Input: part model. Units: mm. Frame: model coordinates. A direction names the side the tool comes from. Give positions to 0.01 mm unless a question says otherwise; leave off trailing zeros. Write each loop counter-clockwise with the first axis right and the second up, starting at its lowest first coordinate (ties: lowest second). Pieces come first, ordered by that corner, then holes. Notation, with made-up numbers: (75.5, 51.25) - (97.5, 51.25) arc R16 cw to (97.5, 60.25) - close; hole circle Ø4 at (-14.75, 69.5). An arc over 180 degrees is marked (long way). Answer as a JSON object with one key per item and string values. Group by question number.
from build123d import *

# Parameters (mm, degrees)
BOSS_EXTRUDE1_OUTLINE_R = 67.5
BOSS_EXTRUDE1_DEPTH     = 35
SKETCH2_R               = 2.5
CUT_EXTRUDE2_DEPTH      = 18
SKETCH4_R               = 25
BOSS_EXTRUDE3_DEPTH     = 35
CUT_EXTRUDE4_DEPTH      = 18
CUT_EXTRUDE7_DEPTH      = 2
CUT_EXTRUDE8_DEPTH      = 30
SKETCH9_R               = 3.5
CUT_EXTRUDE9_DEPTH      = 1


# Read off the part's stored shape, not the designer's step: Boss-Extrude1
with BuildPart() as part:
    # Boss-Extrude1 outline → Boss-Extrude1 (new body)
    with BuildSketch(Plane(origin=(0, 0, 0), x_dir=(1, 0, 0), z_dir=(0, 1, 0))):
        Circle(BOSS_EXTRUDE1_OUTLINE_R)
        with BuildLine():
            ThreePointArc((-13.30331837, -14.257339175), (-10.833619544, -16.21365744), (-8.081104316, -17.746711048))
            Line((-8.081104316, -17.746711048), (-25.687679516, -60.252743681))
            ThreePointArc((-25.687679516, -60.252743681), (-36.389850263, -54.461259606), (-45.836027298, -46.790048103))
            Line((-45.836027298, -46.790048103), (-13.30331837, -14.257339175))
        make_face(mode=Mode.SUBTRACT)
        with BuildLine():
            ThreePointArc((-6.834616064, -18.263023388), (-3.804261279, -19.125312968), (-0.674594581, -19.488327844))
            Line((-0.674594581, -19.488327844), (-0.674594581, -65.496526031))
            ThreePointArc((-0.674594581, -65.496526031), (-12.778416092, -64.241435866), (-24.441191264, -60.76905602))
            Line((-24.441191264, -60.76905602), (-6.834616064, -18.263023388))
        make_face(mode=Mode.SUBTRACT)
        with BuildLine():
            ThreePointArc((-17.746711048, -8.081104316), (-16.21365744, -10.833619544), (-14.257339175, -13.30331837))
            Line((-14.257339175, -13.30331837), (-46.790048103, -45.836027298))
            ThreePointArc((-46.790048103, -45.836027298), (-54.461259606, -36.389850263), (-60.252743681, -25.687679516))
            Line((-60.252743681, -25.687679516), (-17.746711048, -8.081104316))
        make_face(mode=Mode.SUBTRACT)
        with BuildLine():
            ThreePointArc((-19.488327844, -0.674594581), (-19.125312968, -3.804261279), (-18.263023388, -6.834616064))
            Line((-18.263023388, -6.834616064), (-60.76905602, -24.441191264))
            ThreePointArc((-60.76905602, -24.441191264), (-64.241435866, -12.778416092), (-65.496526031, -0.674594581))
            Line((-65.496526031, -0.674594581), (-19.488327844, -0.674594581))
        make_face(mode=Mode.SUBTRACT)
        with BuildLine():
            ThreePointArc((0.674594581, -19.488327844), (3.804261279, -19.125312968), (6.834616064, -18.263023388))
            Line((6.834616064, -18.263023388), (24.441191264, -60.76905602))
            ThreePointArc((24.441191264, -60.76905602), (12.778416092, -64.241435866), (0.674594581, -65.496526031))
            Line((0.674594581, -65.496526031), (0.674594581, -19.488327844))
        make_face(mode=Mode.SUBTRACT)
        with BuildLine():
            ThreePointArc((8.081104316, -17.746711048), (10.833619544, -16.21365744), (13.30331837, -14.257339175))
            Line((13.30331837, -14.257339175), (45.836027298, -46.790048103))
            ThreePointArc((45.836027298, -46.790048103), (36.389850263, -54.461259606), (25.687679516, -60.252743681))
            Line((25.687679516, -60.252743681), (8.081104316, -17.746711048))
        make_face(mode=Mode.SUBTRACT)
        with BuildLine():
            ThreePointArc((14.257339175, -13.30331837), (16.21365744, -10.833619544), (17.746711048, -8.081104316))
            Line((17.746711048, -8.081104316), (60.252743681, -25.687679516))
            ThreePointArc((60.252743681, -25.687679516), (54.461259606, -36.389850263), (46.790048103, -45.836027298))
            Line((46.790048103, -45.836027298), (14.257339175, -13.30331837))
        make_face(mode=Mode.SUBTRACT)
        with BuildLine():
            ThreePointArc((18.263023388, -6.834616064), (19.125312968, -3.804261279), (19.488327844, -0.674594581))
            Line((19.488327844, -0.674594581), (65.496526031, -0.674594581))
            ThreePointArc((65.496526031, -0.674594581), (64.241435866, -12.778416092), (60.76905602, -24.441191264))
            Line((60.76905602, -24.441191264), (18.263023388, -6.834616064))
        make_face(mode=Mode.SUBTRACT)
        with BuildLine():
            ThreePointArc((-18.263023388, 6.834616064), (-19.125312968, 3.804261279), (-19.488327844, 0.674594581))
            Line((-19.488327844, 0.674594581), (-65.496526031, 0.674594581))
            ThreePointArc((-65.496526031, 0.674594581), (-64.241435866, 12.778416092), (-60.76905602, 24.441191264))
            Line((-60.76905602, 24.441191264), (-18.263023388, 6.834616064))
        make_face(mode=Mode.SUBTRACT)
        with BuildLine():
            ThreePointArc((-14.257339175, 13.30331837), (-16.21365744, 10.833619544), (-17.746711048, 8.081104316))
            Line((-17.746711048, 8.081104316), (-60.252743681, 25.687679516))
            ThreePointArc((-60.252743681, 25.687679516), (-54.461259606, 36.389850263), (-46.790048103, 45.836027298))
            Line((-46.790048103, 45.836027298), (-14.257339175, 13.30331837))
        make_face(mode=Mode.SUBTRACT)
        with BuildLine():
            ThreePointArc((-8.081104316, 17.746711048), (-10.833619544, 16.21365744), (-13.30331837, 14.257339175))
            Line((-13.30331837, 14.257339175), (-45.836027298, 46.790048103))
            ThreePointArc((-45.836027298, 46.790048103), (-36.389850263, 54.461259606), (-25.687679516, 60.252743681))
            Line((-25.687679516, 60.252743681), (-8.081104316, 17.746711048))
        make_face(mode=Mode.SUBTRACT)
        with BuildLine():
            Line((-6.834616064, 18.263023388), (-24.441191264, 60.76905602))
            ThreePointArc((-24.441191264, 60.76905602), (-12.778416092, 64.241435866), (-0.674594581, 65.496526031))
            Line((-0.674594581, 65.496526031), (-0.674594581, 19.488327844))
            ThreePointArc((-0.674594581, 19.488327844), (-3.804261279, 19.125312968), (-6.834616064, 18.263023388))
        make_face(mode=Mode.SUBTRACT)
        with BuildLine():
            ThreePointArc((19.488327844, 0.674594581), (19.125312968, 3.804261279), (18.263023388, 6.834616064))
            Line((18.263023388, 6.834616064), (60.76905602, 24.441191264))
            ThreePointArc((60.76905602, 24.441191264), (64.241435866, 12.778416092), (65.496526031, 0.674594581))
            Line((65.496526031, 0.674594581), (19.488327844, 0.674594581))
        make_face(mode=Mode.SUBTRACT)
        with BuildLine():
            ThreePointArc((17.746711048, 8.081104316), (16.21365744, 10.833619544), (14.257339175, 13.30331837))
            Line((14.257339175, 13.30331837), (46.790048103, 45.836027298))
            ThreePointArc((46.790048103, 45.836027298), (54.461259606, 36.389850263), (60.252743681, 25.687679516))
            Line((60.252743681, 25.687679516), (17.746711048, 8.081104316))
        make_face(mode=Mode.SUBTRACT)
        with BuildLine():
            ThreePointArc((6.834616064, 18.263023388), (3.804261279, 19.125312968), (0.674594581, 19.488327844))
            Line((0.674594581, 19.488327844), (0.674594581, 65.496526031))
            ThreePointArc((0.674594581, 65.496526031), (12.778416092, 64.241435866), (24.441191264, 60.76905602))
            Line((24.441191264, 60.76905602), (6.834616064, 18.263023388))
        make_face(mode=Mode.SUBTRACT)
        with BuildLine():
            ThreePointArc((13.30331837, 14.257339175), (10.833619544, 16.21365744), (8.081104316, 17.746711048))
            Line((8.081104316, 17.746711048), (25.687679516, 60.252743681))
            ThreePointArc((25.687679516, 60.252743681), (36.389850263, 54.461259606), (45.836027298, 46.790048103))
            Line((45.836027298, 46.790048103), (13.30331837, 14.257339175))
        make_face(mode=Mode.SUBTRACT)
    extrude(amount=BOSS_EXTRUDE1_DEPTH)

    # Sketch2 → Cut-Extrude2 (cut)
    with BuildSketch(Plane.XZ):
        with Locations(Location((0, 0, 0), (0, 0, 270))):
            Circle(SKETCH2_R)
    extrude(amount=-CUT_EXTRUDE2_DEPTH, mode=Mode.SUBTRACT)

    # Sketch4 → Boss-Extrude3 (add)
    with BuildSketch(Plane(origin=(0, 0, 0), x_dir=(1, 0, 0), z_dir=(0, 1, 0))):
        Circle(SKETCH4_R)
    extrude(amount=BOSS_EXTRUDE3_DEPTH)

    # Sketch5 → Cut-Extrude4 (cut)
    with BuildSketch(Plane.XZ):
        with BuildLine():
            Line((-1.5, 2), (1.5, 2))
            ThreePointArc((1.5, 2), (0, -2.5), (-1.5, 2))
        make_face()
    extrude(amount=-CUT_EXTRUDE4_DEPTH, mode=Mode.SUBTRACT)

    # Sketch6 → Cut-Extrude7 (cut)
    with BuildSketch(Plane.XZ):
        with BuildLine():
            Line((-7.714466094, 14.785533906), (0, 7.071067812))
            Line((0, 7.071067812), (7.714466094, 14.785533906))
            Line((7.714466094, 14.785533906), (11.976558152, 19.047625963))
            ThreePointArc((11.976558152, 19.047625963), (15.909902577, 15.909902577), (19.047625963, 11.976558152))
            Line((19.047625963, 11.976558152), (14.785533906, 7.714466094))
            Line((14.785533906, 7.714466094), (7.071067812, 0))
            Line((7.071067812, 0), (14.785533906, -7.714466094))
            Line((14.785533906, -7.714466094), (19.047625963, -11.976558152))
            ThreePointArc((19.047625963, -11.976558152), (15.909902577, -15.909902577), (11.976558152, -19.047625963))
            Line((11.976558152, -19.047625963), (7.714466094, -14.785533906))
            Line((7.714466094, -14.785533906), (0, -7.071067812))
            Line((0, -7.071067812), (-7.714466094, -14.785533906))
            Line((-7.714466094, -14.785533906), (-11.976558152, -19.047625963))
            ThreePointArc((-11.976558152, -19.047625963), (-15.909902577, -15.909902577), (-19.047625963, -11.976558152))
            Line((-19.047625963, -11.976558152), (-14.785533906, -7.714466094))
            Line((-14.785533906, -7.714466094), (-7.071067812, 0))
            Line((-7.071067812, 0), (-14.785533906, 7.714466094))
            Line((-14.785533906, 7.714466094), (-19.047625963, 11.976558152))
            ThreePointArc((-19.047625963, 11.976558152), (-15.909902577, 15.909902577), (-11.976558152, 19.047625963))
            Line((-11.976558152, 19.047625963), (-7.714466094, 14.785533906))
        make_face()
    extrude(amount=-CUT_EXTRUDE7_DEPTH, mode=Mode.SUBTRACT)

    # Sketch7 → Cut-Extrude8 (cut)
    with BuildSketch(Plane.XZ):
        with BuildLine():
            Line((9.899494937, 0), (20.070097993, 10.170603057))
            ThreePointArc((20.070097993, 10.170603057), (22.5, 0), (20.070097993, -10.170603057))
            Line((20.070097993, -10.170603057), (9.899494937, 0))
        make_face()
        with BuildLine():
            Line((0, 9.899494937), (-10.170603057, 20.070097993))
            ThreePointArc((-10.170603057, 20.070097993), (0, 22.5), (10.170603057, 20.070097993))
            Line((10.170603057, 20.070097993), (0, 9.899494937))
        make_face()
        with BuildLine():
            Line((0, -9.899494937), (10.170603057, -20.070097993))
            ThreePointArc((10.170603057, -20.070097993), (0, -22.5), (-10.170603057, -20.070097993))
            Line((-10.170603057, -20.070097993), (0, -9.899494937))
        make_face()
        with BuildLine():
            Line((-9.899494937, 0), (-20.070097993, -10.170603057))
            ThreePointArc((-20.070097993, -10.170603057), (-22.5, 0), (-20.070097993, 10.170603057))
            Line((-20.070097993, 10.170603057), (-9.899494937, 0))
        make_face()
    extrude(amount=-CUT_EXTRUDE8_DEPTH, mode=Mode.SUBTRACT)

    # Sketch9 → Cut-Extrude9 (cut)
    with BuildSketch(Plane(origin=(0, 2, 0), x_dir=(-1, 0, 0), z_dir=(0, -1, 0))):
        with Locations(Location((0, 0, 0), (0, 0, 90))):
            Circle(SKETCH9_R)
    extrude(amount=-CUT_EXTRUDE9_DEPTH, mode=Mode.SUBTRACT)


solid = part.part
1) Reachability of faces 1 (the face through (54.366, 17.255, -36.532)), 2 (the face through (-18, 30, 0)) from +Z, -Z, +X, -X, +Y, -Y: full face, straight path, thin tool, end or side. Return the list, or none.
2) Cut plane D-D on y = 15.5. Count the separate pieces of the cut face and the enclosed holes in it, and give its area (3 significant figures).
3) Pin query (flat end, axial travel): P1, Ø10.5, axis at y = 13, z = 43.5, coming from the +X side; P2, Ø17.5, axis at y = 21.5, z = -49, coming from the +X side; P3, Ø6, axis at x = 0, z = 0, coming from the -Y side; P4, Ø12, axis at y = 3.5, z = 0.5, coming from the -X side. Return the tip coordinate at first contact, or that it passes through.
4) Cut plane B-B on z = -42. Return the cut outline in (x, y).
5) Cut plane A-A on x = -49. Return the cut outline in (y, z).
6) Cut plane C-C on x = 44. Return the cut outline in (y, z), and give its area (3 significant figures).
7) Line query: line 1 along Z through (x, y) = (0, 7.5); line 2 along X through (y, z) = (2.4, 0); line 3 along X through (y, z) = (14.5, 0). Output: solid intervals per line, ascending. Write a range as from..to.
8) Mould query, pull axis X, two halves, no side actions, for faces 3 (the face through (-0.3, 0, 9.7)), 4 (the face through (-64.275, 17.255, -12.611)), 5 (the face through (-4.82, 17.26, -24.53)). Classes: +X half, -X half, draft (parallel to the pull), parting line (faces both ways), or undercut.
Filled in:
{
 "1": {"face 1": "+Y, -Y", "face 2": "-Y"},
 "2": {"separate pieces": "1", "enclosed holes": "21", "area": "3,110 mm²"},
 "3": {"P1": "stops at x = 55.62", "P2": "stops at x = 54.19", "P3": "stops at y = 3", "P4": "stops at x = -67.5"},
 "4": {"outline": "(-52.84, 0) - (-50.26, 0) - (-50.26, 35) - (-52.84, 35) - close; (-42.95, 0) - (-41.05, 0) - (-41.05, 35) - (-42.95, 35) - close; (-18.13, 0) - (-16.67, 0) - (-16.67, 35) - (-18.13, 35) - close; (-0.67, 0) - (0.67, 0) - (0.67, 35) - (-0.67, 35) - close; (16.67, 0) - (18.13, 0) - (18.13, 35) - (16.67, 35) - close; (41.05, 0) - (42.95, 0) - (42.95, 35) - (41.05, 35) - close; (50.26, 0) - (52.84, 0) - (52.84, 35) - (50.26, 35) - close"},
 "5": {"outline": "(0, -46.42) - (35, -46.42) - (35, -43.47) - (0, -43.47) - close; (0, -21.03) - (35, -21.03) - (35, -19.57) - (0, -19.57) - close; (0, -0.67) - (35, -0.67) - (35, 0.67) - (0, 0.67) - close; (0, 19.57) - (35, 19.57) - (35, 21.03) - (0, 21.03) - close; (0, 43.47) - (35, 43.47) - (35, 46.42) - (0, 46.42) - close"},
 "6": {"outline": "(0, -51.19) - (35, -51.19) - (35, -48.52) - (0, -48.52) - close; (0, -44.95) - (35, -44.95) - (35, -43.05) - (0, -43.05) - close; (0, -18.96) - (35, -18.96) - (35, -17.5) - (0, -17.5) - close; (0, -0.67) - (35, -0.67) - (35, 0.67) - (0, 0.67) - close; (0, 17.5) - (35, 17.5) - (35, 18.96) - (0, 18.96) - close; (0, 43.05) - (35, 43.05) - (35, 44.95) - (0, 44.95) - close; (0, 48.52) - (35, 48.52) - (35, 51.19) - (0, 51.19) - close", "area": "470 mm²"},
 "7": {"line 1": "z = -67.5..-22.5, -9.9..-2.5, 2..9.9, 22.5..67.5", "line 2": "x = -67.5..-22.5, -9.9..-3.5, 3.5..9.9, 22.5..67.5", "line 3": "x = -67.5..-22.5, -9.9..-2.5, 2.5..9.9, 22.5..67.5"},
 "8": {"face 3": "draft", "face 4": "undercut", "face 5": "undercut"}
}
